Design review of the part built by this model. Coordinates are the model's own, in mm. A direction names the side the tool comes from. Round coordinates to 2 decimals unless told otherwise and drop trailing zeros. Write each loop counter-clockwise with the first axis right and the second up, starting at its lowest first coordinate (ties: lowest second). Pieces come first, ordered by that corner, then holes. Notation, with made-up numbers: M 62.25,6.25 L 90.25,6.25 A24 ccw 90.25,23.25 Z; hole C 89,63 d9. An arc over 180 degrees is marked long. Use CSV: the item, a comma, the result in double quotes.
from build123d import *

# Parameters (mm, degrees)
EXTRUDE_1_DEPTH     = 106
SKETCH_4_R          = 1.75
EXTRUDE_2_DEPTH     = 34.6
SKETCH_5_R          = 1.75
EXTRUDE_3_DEPTH     = 40.6
SKETCH_8_W          = 30
SKETCH_8_H          = 60
EXTRUDE_4_DEPTH     = 3.5
SKETCH_9_W          = 26
SKETCH_9_H          = 51
CUT_EXTRUDE_1_DEPTH = 1.5
SKETCH_10_W         = 17
SKETCH_10_H         = 51
CUT_EXTRUDE_2_DEPTH = 2
CUT_EXTRUDE_4_REACH = 152.505
SKETCH_11_W         = 14
SKETCH_11_H         = 50
FILLET_3_R          = 1
FILLET_4_R          = 1
SKETCH_13_W         = 51
SKETCH_13_H         = 76
EXTRUDE_5_DEPTH     = 3.5
SKETCH_14_W         = 50
SKETCH_14_H         = 72
CUT_EXTRUDE_5_DEPTH = 2
CUT_EXTRUDE_7_REACH = 156.192
SKETCH_15_R         = 4.5
SKETCH_15_W         = 8
SKETCH_15_H         = 8


with BuildPart() as part:
    # Sketch 2 → Extrude 1 (new body)
    with BuildSketch(Plane.XY):
        Polygon((0, 0), (55, 0), (84.393876913, 6), (106, 6), (106, 4.5), (84.393876913, 4.5), (55, -1.5), (0, -1.5), align=None)
    extrude(amount=EXTRUDE_1_DEPTH)

    # Sketch 4 → Extrude 2 (add)
    with BuildSketch(Plane.XZ.offset(1.5)):
        with Locations(Location((4.5, 101.5, 0), (0, 0, 180))):
            Circle(SKETCH_4_R)
    extrude_2 = extrude(amount=EXTRUDE_2_DEPTH)

    # Sketch 5 → Extrude 3 (add)
    with BuildSketch(Plane.XZ.offset(-4.5)):
        with Locations(Location((101.5, 101.5, 0), (0, 0, 180))):
            Circle(SKETCH_5_R)
    extrude_3 = extrude(amount=EXTRUDE_3_DEPTH)

    # Mirror 1: Extrude 2, Extrude 3 across plane
    add(extrude_2.mirror(Plane.XY.offset(53)))
    add(extrude_3.mirror(Plane.XY.offset(53)))

    # Sketch 8 → Extrude 4 (add)
    with BuildSketch(Plane(origin=(2.493938769, -12.217754868, 0), x_dir=(0.9797958971132713, 0.20000000000000007, 0), z_dir=(0.20000000000000007, -0.9797958971132713, 0))):
        with Locations((68.588774341, 53)):
            Rectangle(SKETCH_8_W, SKETCH_8_H)
    extrude(amount=EXTRUDE_4_DEPTH)

    # Sketch 9 → Cut-Extrude 1 (cut)
    with BuildSketch(Plane(origin=(3.193938769, -15.647040508, 0), x_dir=(0.9797958971132713, 0.19999999999999998, 0), z_dir=(0.19999999999999998, -0.9797958971132713, 0))):
        with Locations((68.588774341, 53)):
            Rectangle(SKETCH_9_W, SKETCH_9_H)
    extrude(amount=-CUT_EXTRUDE_1_DEPTH, mode=Mode.SUBTRACT)

    # Sketch 10 → Cut-Extrude 2 (cut)
    with BuildSketch(Plane(origin=(2.893938769, -14.177346662, 0), x_dir=(0.9797958971132713, 0.19999999999999998, 0), z_dir=(0.19999999999999998, -0.9797958971132713, 0))):
        with Locations((69.088774341, 53)):
            Rectangle(SKETCH_10_W, SKETCH_10_H)
    extrude(amount=-CUT_EXTRUDE_2_DEPTH, mode=Mode.SUBTRACT)

    # Sketch 11 → Cut-Extrude 4 (cut, up to next)
    with BuildSketch(Plane(origin=(2.2, -10.777754868, 0), x_dir=(0.9797958971132713, 0.20000000000000007, 0), z_dir=(-0.20000000000000007, 0.9797958971132713, 0)), mode=Mode.PRIVATE) as cut_extrude_4_sk1:
        with Locations((70.588774341, -53)):
            Rectangle(SKETCH_11_W, SKETCH_11_H)
    cut_extrude_4_tool1 = extrude(cut_extrude_4_sk1.sketch, amount=-CUT_EXTRUDE_4_REACH, mode=Mode.PRIVATE) & part.part
    add(cut_extrude_4_tool1.solids().sort_by_distance((71.362591, 3.34, 53))[0], mode=Mode.SUBTRACT)

    # Fillet 3
    fillet_3_edges = [part.edges().sort_by_distance(p)[0] for p in [
        (0, 0, 53),
        (55, 0, 53),
        (84.393876913, 6, 53),
        (106, 6, 53),
        (95.196938457, 6, 106),
        (69.696938457, 3, 106),
        (27.5, 0, 106),
        (27.5, 0, 0),
        (69.696938457, 3, 0),
        (95.196938457, 6, 0),
        (64.504020202, 1.94, 53),
        (71.362591482, 3.34, 78),
        (78.221162762, 4.74, 53),
        (71.362591482, 3.34, 28),
    ]]
    fillet(fillet_3_edges, radius=FILLET_3_R)

    # Fillet 4
    fillet_4_edges = [part.edges().sort_by_distance(p)[0] for p in [
        (69.696938457, 1.5, 23),
        (69.696938457, 1.5, 83),
        (55.7, -4.92928564, 53),
        (70.396938457, -1.92928564, 23),
        (85.093876913, 1.07071436, 53),
        (70.396938457, -1.92928564, 83),
    ]]
    fillet(fillet_4_edges, radius=FILLET_4_R)

    # Sketch 13 → Extrude 5 (add)
    with BuildSketch(Plane.XZ.offset(1.5)):
        with Locations((27.5, 53)):
            Rectangle(SKETCH_13_W, SKETCH_13_H)
    extrude(amount=EXTRUDE_5_DEPTH)

    # Sketch 14 → Cut-Extrude 5 (cut)
    with BuildSketch(Plane.XZ.offset(5)):
        with Locations((28, 53)):
            Rectangle(SKETCH_14_W, SKETCH_14_H)
    extrude(amount=-CUT_EXTRUDE_5_DEPTH, mode=Mode.SUBTRACT)

    # Sketch 15 → Cut-Extrude 7 (cut, up to next)
    with BuildSketch(Plane(origin=(0, 0, 0), x_dir=(1, 0, 0), z_dir=(0, 1, 0)), mode=Mode.PRIVATE) as cut_extrude_7_sk1:
        with Locations(Location((29, -36, 0), (0, 0, 270))):
            Circle(SKETCH_15_R)
    cut_extrude_7_tool1 = extrude(cut_extrude_7_sk1.sketch, amount=-CUT_EXTRUDE_7_REACH, mode=Mode.PRIVATE) & part.part
    # Sketch 15 → Cut-Extrude 7 (cut, up to next)
    with BuildSketch(Plane(origin=(0, 0, 0), x_dir=(1, 0, 0), z_dir=(0, 1, 0)), mode=Mode.PRIVATE) as cut_extrude_7_sk2:
        with Locations(Location((38.5, -26.5, 0), (0, 0, 270))):
            Circle(SKETCH_15_R)
    cut_extrude_7_tool2 = extrude(cut_extrude_7_sk2.sketch, amount=-CUT_EXTRUDE_7_REACH, mode=Mode.PRIVATE) & part.part
    # Sketch 15 → Cut-Extrude 7 (cut, up to next)
    with BuildSketch(Plane(origin=(0, 0, 0), x_dir=(1, 0, 0), z_dir=(0, 1, 0)), mode=Mode.PRIVATE) as cut_extrude_7_sk3:
        with Locations(Location((38.5, -45.5, 0), (0, 0, 270))):
            Circle(SKETCH_15_R)
    cut_extrude_7_tool3 = extrude(cut_extrude_7_sk3.sketch, amount=-CUT_EXTRUDE_7_REACH, mode=Mode.PRIVATE) & part.part
    # Sketch 15 → Cut-Extrude 7 (cut, up to next)
    with BuildSketch(Plane(origin=(0, 0, 0), x_dir=(1, 0, 0), z_dir=(0, 1, 0)), mode=Mode.PRIVATE) as cut_extrude_7_sk4:
        with Locations(Location((19.5, -26.5, 0), (0, 0, 270))):
            Circle(SKETCH_15_R)
    cut_extrude_7_tool4 = extrude(cut_extrude_7_sk4.sketch, amount=-CUT_EXTRUDE_7_REACH, mode=Mode.PRIVATE) & part.part
    # Sketch 15 → Cut-Extrude 7 (cut, up to next)
    with BuildSketch(Plane(origin=(0, 0, 0), x_dir=(1, 0, 0), z_dir=(0, 1, 0)), mode=Mode.PRIVATE) as cut_extrude_7_sk5:
        with Locations(Location((19.5, -45.5, 0), (0, 0, 270))):
            Circle(SKETCH_15_R)
    cut_extrude_7_tool5 = extrude(cut_extrude_7_sk5.sketch, amount=-CUT_EXTRUDE_7_REACH, mode=Mode.PRIVATE) & part.part
    # Sketch 15 → Cut-Extrude 7 (cut, up to next)
    with BuildSketch(Plane(origin=(0, 0, 0), x_dir=(1, 0, 0), z_dir=(0, 1, 0)), mode=Mode.PRIVATE) as cut_extrude_7_sk6:
        with Locations((39, -36)):
            Rectangle(SKETCH_15_W, SKETCH_15_H)
    cut_extrude_7_tool6 = extrude(cut_extrude_7_sk6.sketch, amount=-CUT_EXTRUDE_7_REACH, mode=Mode.PRIVATE) & part.part
    # Sketch 15 → Cut-Extrude 7 (cut, up to next)
    with BuildSketch(Plane(origin=(0, 0, 0), x_dir=(1, 0, 0), z_dir=(0, 1, 0)), mode=Mode.PRIVATE) as cut_extrude_7_sk7:
        with Locations((29, -26)):
            Rectangle(SKETCH_15_W, SKETCH_15_H)
    cut_extrude_7_tool7 = extrude(cut_extrude_7_sk7.sketch, amount=-CUT_EXTRUDE_7_REACH, mode=Mode.PRIVATE) & part.part
    # Sketch 15 → Cut-Extrude 7 (cut, up to next)
    with BuildSketch(Plane(origin=(0, 0, 0), x_dir=(1, 0, 0), z_dir=(0, 1, 0)), mode=Mode.PRIVATE) as cut_extrude_7_sk8:
        with Locations((29, -46)):
            Rectangle(SKETCH_15_W, SKETCH_15_H)
    cut_extrude_7_tool8 = extrude(cut_extrude_7_sk8.sketch, amount=-CUT_EXTRUDE_7_REACH, mode=Mode.PRIVATE) & part.part
    # Sketch 15 → Cut-Extrude 7 (cut, up to next)
    with BuildSketch(Plane(origin=(0, 0, 0), x_dir=(1, 0, 0), z_dir=(0, 1, 0)), mode=Mode.PRIVATE) as cut_extrude_7_sk9:
        with Locations((19, -36)):
            Rectangle(SKETCH_15_W, SKETCH_15_H)
    cut_extrude_7_tool9 = extrude(cut_extrude_7_sk9.sketch, amount=-CUT_EXTRUDE_7_REACH, mode=Mode.PRIVATE) & part.part
    cut_extrude_7_1 = cut_extrude_7_tool1.solids().sort_by_distance((29, 0, 36))[0]
    add(cut_extrude_7_1, mode=Mode.SUBTRACT)
    cut_extrude_7_2 = cut_extrude_7_tool2.solids().sort_by_distance((38.5, 0, 26.5))[0]
    add(cut_extrude_7_2, mode=Mode.SUBTRACT)
    cut_extrude_7_3 = cut_extrude_7_tool3.solids().sort_by_distance((38.5, 0, 45.5))[0]
    add(cut_extrude_7_3, mode=Mode.SUBTRACT)
    cut_extrude_7_4 = cut_extrude_7_tool4.solids().sort_by_distance((19.5, 0, 26.5))[0]
    add(cut_extrude_7_4, mode=Mode.SUBTRACT)
    cut_extrude_7_5 = cut_extrude_7_tool5.solids().sort_by_distance((19.5, 0, 45.5))[0]
    add(cut_extrude_7_5, mode=Mode.SUBTRACT)
    cut_extrude_7_6 = cut_extrude_7_tool6.solids().sort_by_distance((39, 0, 36))[0]
    add(cut_extrude_7_6, mode=Mode.SUBTRACT)
    cut_extrude_7_7 = cut_extrude_7_tool7.solids().sort_by_distance((29, 0, 26))[0]
    add(cut_extrude_7_7, mode=Mode.SUBTRACT)
    cut_extrude_7_8 = cut_extrude_7_tool8.solids().sort_by_distance((29, 0, 46))[0]
    add(cut_extrude_7_8, mode=Mode.SUBTRACT)
    cut_extrude_7_9 = cut_extrude_7_tool9.solids().sort_by_distance((19, 0, 36))[0]
    add(cut_extrude_7_9, mode=Mode.SUBTRACT)
    cut_extrude_7 = cut_extrude_7_1 + cut_extrude_7_2 + cut_extrude_7_3 + cut_extrude_7_4 + cut_extrude_7_5 + cut_extrude_7_6 + cut_extrude_7_7 + cut_extrude_7_8 + cut_extrude_7_9  # Cut-Extrude 7 as one shape, for the pattern or mirror that repeats it

    # Mirror 2: Cut-Extrude 7 across plane
    add(cut_extrude_7.mirror(Plane.XY.offset(53)), mode=Mode.SUBTRACT)


solid = part.part
1) Add section A-A on y = -12. Write out the cut boundary in (x, z).
Answers:
outline,"C 4.5,4.5 d3.5; C 4.5,101.5 d3.5; C 101.5,4.5 d3.5; C 101.5,101.5 d3.5"
2) Add section D-D on x = 49. Write out the cut boundary in (y, z), then the cut area to 3 significant figures.
Answers:
outline,"M -5,15 L -1.5,15 L -1.5,0 L -1,0 A1 ccw 0,1 L 0,105 A1 ccw -1,106 L -1.5,106 L -1.5,91 L -5,91 L -5,89 L -3,89 L -3,17 L -5,17 Z"
area,"281 mm²"
3) Add section B-B on z = 10. Write out the cut boundary in (x, y), then the cut area to 3 significant figures.
Answers:
outline,"M 0,-1.5 L 55,-1.5 L 84.39,4.5 L 106,4.5 L 106,5 A1 ccw 105,6 L 84.49,6 A1 ccw 84.29,5.98 L 55.1,0.02 A1 cw 54.9,0 L 1,0 A1 ccw 0,-1 Z"
area,"159 mm²"
4) Machinability: for faces 1 (the face through (70.543, -1.593, 23.285)), 2 (the face through (28, -3, 54)), 3 (the face through (29, -1, 56)), 4 (the face through (28, 0, 52)), which of the approach directions +Z, -Z, +X, -X, +Y, -Y give a long, thin tool a straight path to every point of the face, cutting with its end or side? Answer none if there is none.
Answers:
face 1,"-Z, +X, -Y"
face 2,"-Y"
face 3,"+Y, -Y"
face 4,"+Z, -Z, -X, +Y"
5) Add section C-C on z = 36. Give the number of separate pieces and of enclosed holes in the cut face, then the cut area to 3 significant figures.
Answers:
separate pieces,"5"
enclosed holes,"0"
area,"173 mm²"
6) The part is to be moulded in two halves that separate along X. For faces 5 (the face through (70, 0, 83)), 6 (the face through (69.96, 2.76, 105.7)), 7 (the face through (27.28, -1.48, 40.16)), say which applies: released by +X, released by -X, zero draft, split by the parting line, or undercut.
Answers:
face 5,"zero draft"
face 6,"released by -X"
face 7,"undercut"
7) For pin 1 Ø3.5 at (x, y) = (17.5, -1) entering from -Z; pin 2 Ø14.5 at (x, z) = (19.5, 79.5) entering from -Y; pin 3 Ø4 at (y, z) = (-3.5, 57.5) entering from +X; pin 4 Ø11 at (x, z) = (92.5, 66) entering from -Y, all flat-tipped, find the tip position at first contact; note any pin that passes through.
Answers:
pin 1,"z = 0"
pin 2,"y = -3"
pin 3,"x = 62.26"
pin 4,"y = 4.5"
8) Wall thickness on line 1 along X through (y, z) = (-1.95, 60.5); line 2 along Y through (x, z) = (9.5, 49); line 3 along Y through (x, z) = (93.5, 47.5): over which ranges is each line inside the solid? List them lowest first. Write a range as [from, to].
Answers:
line 1,"[2, 15], [24, 25], [33, 34], [43, 53], [55.09, 62.24]"
line 2,"[-3, 0]"
line 3,"[4.5, 6]"
